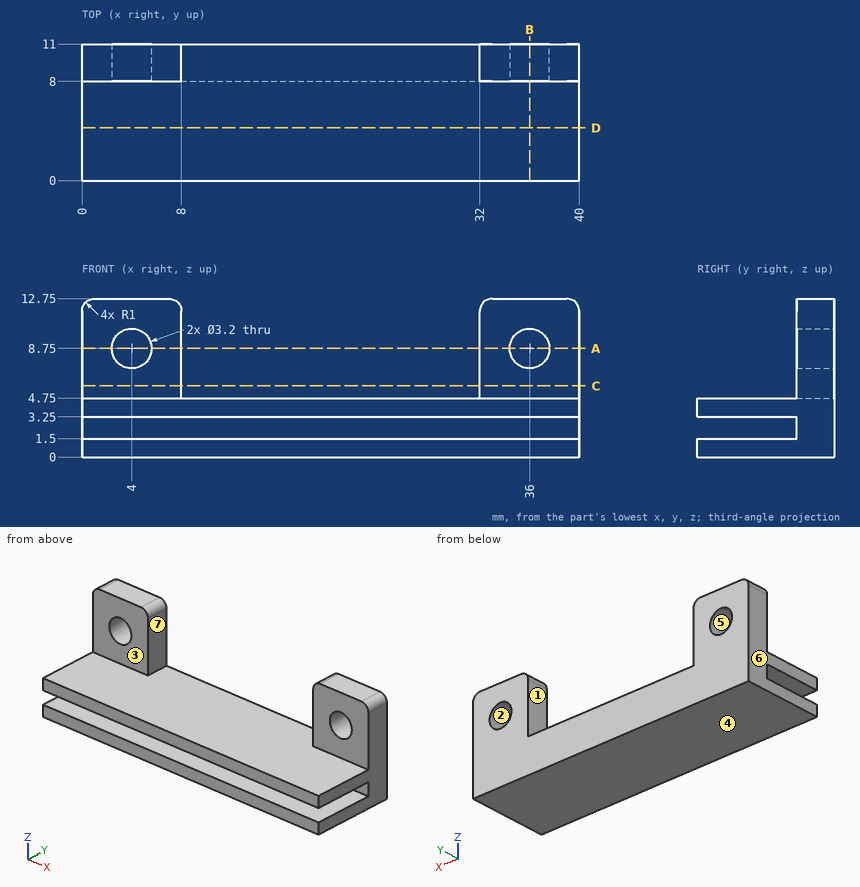
Job drawing, mm, ordinate dimensions from the low corner. One solid piece. A direction names the side the tool comes from. Coordinates: 2 decimals unless noted, no trailing zeros. Write each loop counter-clockwise with the first axis right and the second up, starting at its lowest first coordinate (ties: lowest second). Pieces come first, ordered by that corner, then holes.
Item 1: Which spindle directions (+Z, -Z, +X, -X, +Y, -Y) get a long thin tool onto all of the face, cutting with end or side? Do the marked faces 1, 2 and 3. Say none if no direction does.
Item 2: Mould opens along X. For the marked faces 4, 5, 6 and 7 say: released by +X, released by -X, zero draft, split by the parting line, or undercut.
Item 3: Slice it at A-A (z = 8.75). Write the cut outline in (x, y).
Item 4: Pin check, flat tips, straight feed: pin 1 (6.5 mm diameter, centred on x = 36.5, z = 10, fed in from -Y); pin 2 (2 mm diameter, centred on y = 2, z = 4.5, fed in from -X); pin 3 (6.5 mm diameter, centred on x = 16, y = 4, fed in from +Z). Stop position of each tip, or through.
Item 5: Probe line 1 (Z direction, x = 32.5, y = 2.25); line 2 (X direction, y = 8.25, z = 10); line 3 (X direction, y = 10.75, z = 8). List the from-to ranges inside material, lowest first.
Item 6: Slice it at C-C (z = 5.75). Write the cut outline in (x, y), and give its area (3 significant figures).
Item 7: Slice it at D-D (y = 4.25). Write the cut outline in (x, z), and give its area (3 significant figures).
Item 8: Slice it at B-B (x = 36). Write the cut outline in (y, z), and give its area (4 significant figures).
Results found:
1. face 1: +Z, +Y, -Y
1. face 2: +Y, -Y
1. face 3: +Z, +X, -X, -Y
2. face 4: zero draft
2. face 5: undercut
2. face 6: released by -X
2. face 7: undercut
3. outline: (0, 8) - (2.4, 8) - (2.4, 11) - (0, 11) - close; (5.6, 8) - (8, 8) - (8, 11) - (5.6, 11) - close; (32, 8) - (34.4, 8) - (34.4, 11) - (32, 11) - close; (37.6, 8) - (40, 8) - (40, 11) - (37.6, 11) - close
4. pin 1: stops at y = 8
4. pin 2: stops at x = 0
4. pin 3: stops at z = 4.75
5. line 1: z = 0 to 1.5, 3.25 to 4.75
5. line 2: x = 0 to 3, 5 to 8, 32 to 35, 37 to 40
5. line 3: x = 0 to 2.59, 5.41 to 8, 32 to 34.59, 37.41 to 40
6. outline: (0, 8) - (8, 8) - (8, 11) - (0, 11) - close; (32, 8) - (40, 8) - (40, 11) - (32, 11) - close
6. area: 48.0 mm2
7. outline: (0, 0) - (40, 0) - (40, 1.5) - (0, 1.5) - close; (0, 3.25) - (40, 3.25) - (40, 4.75) - (0, 4.75) - close
7. area: 120 mm2
8. outline: (0, 0) - (11, 0) - (11, 7.15) - (8, 7.15) - (8, 4.75) - (0, 4.75) - (0, 3.25) - (8, 3.25) - (8, 1.5) - (0, 1.5) - close; (8, 10.35) - (11, 10.35) - (11, 12.75) - (8, 12.75) - close
8. area: 52.65 mm2
